from build123d import *

# Parameters (mm, degrees)
SKETCH1_R           = 15
SKETCH1_R_2         = 5.15
BOSS_EXTRUDE1_DEPTH = 1.3
BOSS_EXTRUDE2_START = -1.65
SKETCH1_3_R         = 15
SKETCH1_3_R_2       = 10.75
BOSS_EXTRUDE2_DEPTH = 1.65
CUT_EXTRUDE1_START  = -1.65
CUT_EXTRUDE1_DEPTH  = 1.65
FILLET5_R           = 0.5
FILLET6_R           = 0.5


with BuildPart() as part:
    # Sketch1 → Boss-Extrude1 (new body)
    with BuildSketch(Plane(origin=(0, 0, 0), x_dir=(1, 0, 0), z_dir=(0, 1, 0))):
        with Locations(Location((0, 0, 0), (0, 0, 270))):
            Circle(SKETCH1_R)
        with Locations(Location((-7, 0, 0), (0, 0, 270))):
            Circle(SKETCH1_R_2, mode=Mode.SUBTRACT)
    extrude(amount=BOSS_EXTRUDE1_DEPTH)

    # Sketch1_3 → Boss-Extrude2 (add)
    with BuildSketch(Plane(origin=(0, 0, 0), x_dir=(1, 0, 0), z_dir=(0, 1, 0)).offset(BOSS_EXTRUDE2_START)):
        with Locations(Location((0, 0, 0), (0, 0, 270))):
            Circle(SKETCH1_3_R)
        with Locations(Location((0, 0, 0), (0, 0, 270))):
            Circle(SKETCH1_3_R_2, mode=Mode.SUBTRACT)
    extrude(amount=BOSS_EXTRUDE2_DEPTH)

    # Sketch1_4 → Cut-Extrude1 (cut)
    with BuildSketch(Plane(origin=(0, 0, 0), x_dir=(1, 0, 0), z_dir=(0, 1, 0)).offset(CUT_EXTRUDE1_START)):
        with BuildLine():
            ThreePointArc((-9.86, -4.282861193), (-4.571677534, -4.541558103), (-1.85, 0))
            Line((-1.85, 0), (-10.75, 0))
            ThreePointArc((-10.75, 0), (-10.525148455, -2.187178548), (-9.86, -4.282861193))
        make_face()
        with BuildLine():
            Line((-10.75, 0), (-1.85, 0))
            ThreePointArc((-1.85, 0), (-4.571677534, 4.541558103), (-9.86, 4.282861193))
            ThreePointArc((-9.86, 4.282861193), (-10.525148455, 2.187178548), (-10.75, 0))
        make_face()
        with BuildLine():
            ThreePointArc((-9.86, 4.282861193), (-4.571677534, 4.541558103), (-1.85, 0))
            ThreePointArc((-1.85, 0), (-4.571677534, -4.541558103), (-9.86, -4.282861193))
            ThreePointArc((-9.86, -4.282861193), (2.187178548, -10.525148455), (10.75, 0))
            ThreePointArc((10.75, 0), (2.187178548, 10.525148455), (-9.86, 4.282861193))
        make_face()
        with BuildLine():
            ThreePointArc((-9.86, -4.282861193), (-10.525148455, -2.187178548), (-10.75, 0))
            Line((-10.75, 0), (-12.15, 0))
            ThreePointArc((-12.15, 0), (-11.541558103, -2.428322466), (-9.86, -4.282861193))
        make_face()
        with BuildLine():
            Line((-12.15, 0), (-10.75, 0))
            ThreePointArc((-10.75, 0), (-10.525148455, 2.187178548), (-9.86, 4.282861193))
            ThreePointArc((-9.86, 4.282861193), (-11.541558103, 2.428322466), (-12.15, 0))
        make_face()
    extrude(amount=CUT_EXTRUDE1_DEPTH, mode=Mode.SUBTRACT)

    # Fillet5
    fillet5_edges = [part.edges().sort_by_distance(p)[0] for p in [
        (-7, 1.3, -5.15),
    ]]
    fillet(fillet5_edges, radius=FILLET5_R)

    # Fillet6
    fillet6_edges = [part.edges().sort_by_distance(p)[0] for p in [
        (0, -1.65, -15),
        (10.75, -1.65, 0),
    ]]
    fillet(fillet6_edges, radius=FILLET6_R)


solid = part.part
Source: CAD feature listing. Evaluate the final solid. Frame: model axes, mm. A direction names the side the tool comes from. Round coordinates to 2 decimals unless told otherwise and drop trailing zeros. Loops run counter-clockwise (first coordinate to the right, second up) from the corner with the lowest first, then second, coordinate; pieces in that order, holes last.
Q1. Access query for faces 1 (the face through (3, 0, 0)), 2 (the face through (0, 1.3, 0)). Directions: +Z, -Z, +X, -X, +Y, -Y. A direction counts if a zero-diameter tool reaches every point of the face in a straight line with its end or side. Return the directions, or none.
Q2. First-contact query: P1, Ø6, axis at x = 2, z = 4, coming from the -Y side. Flat tip, straight axial feed; report the tip coordinate or a pass-through.
Q3. Section B-B, the plane x = 0. Return loops of the section in (y, z).
Q4. Mould query, pull axis Z, two halves, no side actions, for faces 3 (the face through (10.742, -0.583, 0.411)), 4 (the face through (-3, -1.65, -11)), 5 (the face through (0.66, 0.058, -14.985)). Classes: pulls with the +Z half, pulls with the -Z half, needs draft (parallel to the pull), parting line crosses it, or undercut.
Q5. Section A-A, the plane y = 0.4. Return loops of the section in (x, z), plus the area to 3 significant figures.
Q6. Ray query, line 1 (X direction, y = -0.65, z = 0); line 2 (X direction, y = 0.45, z = 0); line 3 (Y direction, x = -7.5, z = -6). Return the intervals inside material, ascending.
Solutions:
1. face 1: -Y
1. face 2: +Z, -Z, +X, -X, +Y
2. P1: stops at y = 0
3. outline: (-1.65, -14.5) arc R0.5 ccw to (-1.15, -15) - (1.3, -15) - (1.3, 15) - (-1.15, 15) arc R0.5 ccw to (-1.65, 14.5) - (-1.65, 11.25) arc R0.5 ccw to (-1.15, 10.75) - (0, 10.75) - (0, -10.75) - (-1.15, -10.75) arc R0.5 ccw to (-1.65, -11.25) - close
4. face 3: undercut
4. face 4: needs draft
4. face 5: parting line crosses it
5. outline: circle Ø30 at (0, 0); hole circle Ø10.3 at (-7, 0)
5. area: 624 mm2
6. line 1: x = -15 to -12.15, 10.75 to 15
6. line 2: x = -15 to -12.15, -1.85 to 15
6. line 3: y = 0 to 1.3
